Model file for the job. Use its own axes, mm. Give positions to 0.01 mm unless a question says otherwise; leave off trailing zeros. Loops run counter-clockwise (first coordinate to the right, second up) from the corner with the lowest first, then second, coordinate; pieces in that order, holes last. Notation, with made-up numbers: M -31.5,18 L 9.5,18 A10 ccw 9.5,36 Z; hole C 64.25,27 d2. An arc over 180 degrees is marked long. Answer in a Markdown table with one row per item.
```python
from build123d import *

# Parameters (mm, degrees)
ESQUISSE1_W              = 250
ESQUISSE1_H              = 210
ESQUISSE1_R              = 1.143
ESQUISSE1_R_2            = 1.134386863
BOSS_EXTRU_1_DEPTH       = 3
ESQUISSE2_R              = 2.5
ESQUISSE2_R_2            = 2
ENL_V_MAT_EXTRU_1_DEPTH  = 5
ESQUISSE3_W              = 250
ESQUISSE3_H              = 50
ENL_V_MAT_EXTRU_2_DEPTH  = 5
ESQUISSE10_W             = 80
ESQUISSE10_H             = 75
ENL_V_MAT_EXTRU_7_DEPTH  = 10
ESQUISSE12_R             = 2
ENL_V_MAT_EXTRU_8_DEPTH  = 13
ESQUISSE18_R             = 2
ENL_V_MAT_EXTRU_13_DEPTH = 10
ESQUISSE19_R             = 3.1
ENL_V_MAT_EXTRU_14_DEPTH = 10
ESQUISSE21_R             = 3.1
ENL_V_MAT_EXTRU_16_DEPTH = 10
ENL_V_MAT_EXTRU_17_DEPTH = 10
ENL_V_MAT_EXTRU_18_DEPTH = 10


with BuildPart() as part:
    # Esquisse1 → Boss.-Extru.1 (new body)
    with BuildSketch(Plane.XY):
        with Locations((125, -105)):
            Rectangle(ESQUISSE1_W, ESQUISSE1_H)
        with Locations((94.002297733, -70.627273701)):
            Circle(ESQUISSE1_R, mode=Mode.SUBTRACT)
        with Locations((98.297909971, -84.719098973)):
            Circle(ESQUISSE1_R_2, mode=Mode.SUBTRACT)
    extrude(amount=BOSS_EXTRU_1_DEPTH)

    # Esquisse2 → Enlèv. mat.-Extru.1 (cut)
    with BuildSketch(Plane.XY.offset(3)):
        with Locations((18, -137)):
            Circle(ESQUISSE2_R)
        with Locations((18, -188)):
            Circle(ESQUISSE2_R)
        with Locations((85, -142.5)):
            Circle(ESQUISSE2_R_2)
        with Locations((118.4, -142.5)):
            Circle(ESQUISSE2_R_2)
        with Locations((118.4, -177.5)):
            Circle(ESQUISSE2_R_2)
        with Locations((85, -177.5)):
            Circle(ESQUISSE2_R_2)
        with Locations((131.6, -177.5)):
            Circle(ESQUISSE2_R_2)
        with Locations((165, -177.5)):
            Circle(ESQUISSE2_R_2)
        with Locations((165, -142.5)):
            Circle(ESQUISSE2_R_2)
        with Locations((131.6, -142.5)):
            Circle(ESQUISSE2_R_2)
        with Locations((232, -188)):
            Circle(ESQUISSE2_R)
        with Locations((232, -137)):
            Circle(ESQUISSE2_R)
    extrude(amount=-ENL_V_MAT_EXTRU_1_DEPTH, mode=Mode.SUBTRACT)

    # Esquisse3 → Enlèv. mat.-Extru.2 (cut)
    with BuildSketch(Plane.XY.offset(3)):
        with Locations((125, -25)):
            Rectangle(ESQUISSE3_W, ESQUISSE3_H)
    extrude(amount=-ENL_V_MAT_EXTRU_2_DEPTH, mode=Mode.SUBTRACT)

    # Esquisse10 → Enlèv. mat.-Extru.7 (cut)
    with BuildSketch(Plane.XY.offset(3)):
        with Locations((40, -162.5)):
            Rectangle(ESQUISSE10_W, ESQUISSE10_H)
        with Locations((210, -162.5)):
            Rectangle(ESQUISSE10_W, ESQUISSE10_H)
    extrude(amount=-ENL_V_MAT_EXTRU_7_DEPTH, mode=Mode.SUBTRACT)

    # Esquisse12 → Enlèv. mat.-Extru.8 (cut)
    with BuildSketch(Plane.XY.offset(3)):
        with Locations((39.8, -108.5)):
            Circle(ESQUISSE12_R)
        with Locations((39.8, -70.5)):
            Circle(ESQUISSE12_R)
        with Locations((210.2, -108.5)):
            Circle(ESQUISSE12_R)
        with Locations((210.2, -70.5)):
            Circle(ESQUISSE12_R)
    extrude(amount=-ENL_V_MAT_EXTRU_8_DEPTH, mode=Mode.SUBTRACT)

    # Esquisse18 → Enlèv. mat.-Extru.13 (cut)
    with BuildSketch(Plane.XY.offset(3)):
        with Locations((22, -205)):
            Circle(ESQUISSE18_R)
        with Locations((228, -205)):
            Circle(ESQUISSE18_R)
    extrude(amount=-ENL_V_MAT_EXTRU_13_DEPTH, mode=Mode.SUBTRACT)

    # Esquisse19 → Enlèv. mat.-Extru.14 (cut)
    with BuildSketch(Plane.XY.offset(3)):
        with Locations((90, -117)):
            Circle(ESQUISSE19_R)
        with Locations((90, -202)):
            Circle(ESQUISSE19_R)
        with Locations((160, -202)):
            Circle(ESQUISSE19_R)
        with Locations((160, -117)):
            Circle(ESQUISSE19_R)
    extrude(amount=-ENL_V_MAT_EXTRU_14_DEPTH, mode=Mode.SUBTRACT)

    # Esquisse21 → Enlèv. mat.-Extru.16 (cut)
    with BuildSketch(Plane.XY.offset(3)):
        with Locations((10, -60)):
            Circle(ESQUISSE21_R)
        with Locations((10, -205)):
            Circle(ESQUISSE21_R)
        with Locations((240, -205)):
            Circle(ESQUISSE21_R)
        with Locations((240, -60)):
            Circle(ESQUISSE21_R)
    extrude(amount=-ENL_V_MAT_EXTRU_16_DEPTH, mode=Mode.SUBTRACT)

    # Esquisse23 → Enlèv. mat.-Extru.17 (cut)
    with BuildSketch(Plane.XY.offset(3)):
        with BuildLine():
            Line((15, -50), (0, -50))
            Line((0, -50), (0, -65))
            ThreePointArc((0, -65), (4.393398282, -54.393398282), (15, -50))
        make_face()
        with BuildLine():
            Line((250, -50), (235, -50))
            ThreePointArc((235, -50), (245.606601718, -54.393398282), (250, -65))
            Line((250, -65), (250, -50))
        make_face()
    extrude(amount=-ENL_V_MAT_EXTRU_17_DEPTH, mode=Mode.SUBTRACT)

    # Esquisse24 → Enlèv. mat.-Extru.18 (cut)
    with BuildSketch(Plane.XY.offset(3)):
        with BuildLine():
            Line((30, -50), (105, -50))
            ThreePointArc((105, -50), (67.5, -66.928108612), (30, -50))
        make_face()
        with BuildLine():
            Line((145, -50), (220, -50))
            ThreePointArc((220, -50), (182.5, -66.928108612), (145, -50))
        make_face()
    extrude(amount=-ENL_V_MAT_EXTRU_18_DEPTH, mode=Mode.SUBTRACT)


solid = part.part
```
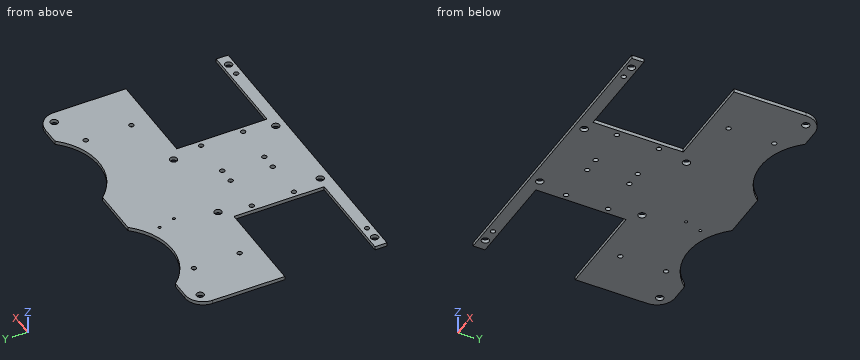
(1) Saw through at C-C, the plane y = -189. Give the cut face in (x, z), and give its area (3 significant figures).
Established:
| item | result |
|---|---|
| outline | M 80,0 L 170,0 L 170,3 L 80,3 Z |
| area | 270 mm2 |
(2) Saw through at B-B, the plane x = 10. Give the cut face in (y, z).
Established:
| item | result |
|---|---|
| outline | M -210,0 L -208.1,0 L -208.1,3 L -210,3 Z; M -201.9,0 L -200,0 L -200,3 L -201.9,3 Z; M -125,0 L -63.1,0 L -63.1,3 L -125,3 Z; M -56.9,0 L -50.86,0 L -50.86,3 L -56.9,3 Z |
(3) Saw through at A-A, the plane x = 178. Give the cut face in (y, z).
Established:
| item | result |
|---|---|
| outline | M -210,0 L -200,0 L -200,3 L -210,3 Z; M -125,0 L -66.73,0 L -66.73,3 L -125,3 Z |
(4) Saw through at D-D, the plane z = 1.9. Count the separate pieces of the cut face and the enclosed holes in it, and give its area (3 significant figures).
Established:
| item | result |
|---|---|
| separate pieces | 1 |
| enclosed holes | 24 |
| area | 25,700 mm2 |
(5) Flat gauge pin, fed straight in: P1, Ø3, axis at x = 210.2, y = -108.5, coming from the +Z side. Where does the tip first touch, or does it go through?
Established:
| item | result |
|---|---|
| P1 | passes through |
(6) Wall check: L1, parallel to Y at x = 131.6, z = 0.8; L2, parallel to X at y = -177.5, z = 1.6; L3, parallel to Y at x = 211.5, z = 0.75. Give the ranges that are in metal, low to high.
Established:
| item | result |
|---|---|
| L1 | y = -210 to -179.5, -175.5 to -144.5, -140.5 to -50 |
| L2 | x = 80 to 83, 87 to 116.4, 120.4 to 129.6, 133.6 to 163, 167 to 170 |
| L3 | y = -210 to -200, -125 to -110.02, -106.98 to -72.02, -68.98 to -57.66 |
